Design review of the part built by this model. Coordinates are the model's own, in mm. Face numbers are marked on the shaded views. A direction names the side the tool comes from. Give positions to 0.01 mm unless a question says otherwise; leave off trailing zeros. One line per item, written item: value.
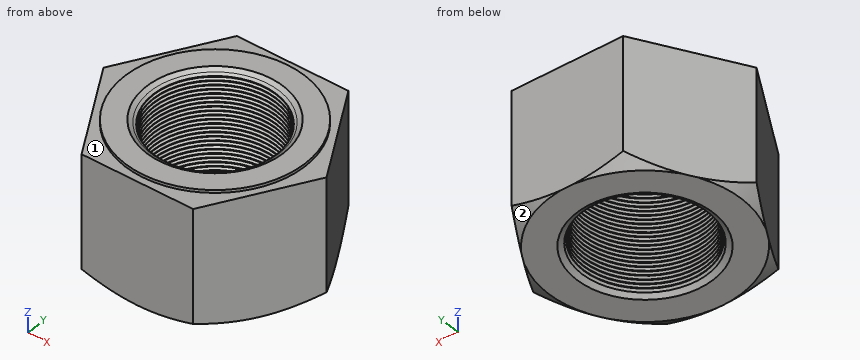
from build123d import *

# Parameters (mm, degrees)
SKETCH1_R         = 17.5
BASENUT_DEPTH     = 34.7
EXTRUDE1_START    = 0.8
SKETCH3_R         = 25.55
SKETCH3_R_2       = 17.5
EXTRUDE1_DEPTH    = 0.8
ENDCHAMFER3_SIZE  = 1.95
ENDCHAMFER3_SIZE2 = 1.125833025
LPATTERN10_COUNT  = 29
LPATTERN10_PITCH  = 1.2


with BuildPart() as part:
    # Sketch1 → BaseNut (new body)
    with BuildSketch(Plane.XY):
        Polygon((15.877132403, -27.5), (31.754264805, 0), (15.877132403, 27.5), (-15.877132403, 27.5), (-31.754264805, 0), (-15.877132403, -27.5), align=None)
        Circle(SKETCH1_R, mode=Mode.SUBTRACT)
    extrude(amount=-BASENUT_DEPTH)

    # Sketch2 → Chamfer1 (revolve, cut)
    with BuildSketch(Plane(origin=(-16.706149795, 0, -15.04811501), x_dir=(0, 0, 1), z_dir=(0, 1, 0))):
        Polygon((-19.65188499, 44.206149795), (-19.65188499, 48.460414601), (-17.195684059, 48.460414601), align=None)
    revolve(axis=Axis((0, 0, -38.770766557), (0, 0, 1)), mode=Mode.SUBTRACT)

    # Sketch6 → EndChamfer1 (revolve, cut)
    with BuildSketch(Plane(origin=(-9.197458863, 0, -10.252541137), x_dir=(0, 0, 1), z_dir=(0, 1, 0))):
        Polygon((-24.447458863, 26.697458863), (-24.447458863, 28.647458863), (-23.321625838, 26.697458863), align=None)
    revolve(axis=Axis((0, 0, 13.104863586), (0, 0, -1)), mode=Mode.SUBTRACT)

    # Sketch3 → Extrude1 (add)
    with BuildSketch(Plane(origin=(-18.48918612, 11.17895969, 0), x_dir=(1, 0, 0), z_dir=(0, 0, 1)).offset(EXTRUDE1_START)):
        with Locations((18.48918612, -11.17895969)):
            Circle(SKETCH3_R)
        with Locations((18.48918612, -11.17895969)):
            Circle(SKETCH3_R_2, mode=Mode.SUBTRACT)
    extrude(amount=-EXTRUDE1_DEPTH)

    # EndChamfer3
    endchamfer3_edges = [part.edges().sort_by_distance(p)[0] for p in [
        (-17.5, 0, 0.8),
    ]]
    endchamfer3_side = [part.faces().sort_by_distance(p)[0] for p in [
        (-24.82733687, 0, 0.8),
    ]]
    chamfer(endchamfer3_edges, length=ENDCHAMFER3_SIZE, length2=ENDCHAMFER3_SIZE2, reference=endchamfer3_side[0])

    # Sketch7 → Cut-Revolve10 (revolve, cut)
    with BuildSketch(Plane(origin=(0, 0, 0), x_dir=(1, 0, 0), z_dir=(0, 1, 0))):
        Polygon((16.5, 34.074166975), (17.5, 34.074166975), (18.366025404, 33.574166975), (17.5, 33.074166975), (16.5, 33.074166975), align=None)
    cut_revolve10 = revolve(axis=Axis((0, 0, -61.609777784), (0, 0, 1)), mode=Mode.SUBTRACT)

    # LPattern10: Cut-Revolve10 ×29
    with Locations(*[(0, 0, i * LPATTERN10_PITCH) for i in range(1, LPATTERN10_COUNT)]):
        add(cut_revolve10, mode=Mode.SUBTRACT)


solid = part.part
Item 1: Clearance check with flat-ended pins moving along their axes: P1, Ø2, axis at y = -17, z = -10.5, coming from the -X side; P2, Ø2, axis at y = -20.5, z = -17.5, coming from the -X side; P3, Ø4, axis at x = 20.5, y = 16.5, coming from the +Z side; P4, Ø6, axis at x = 25, z = -15.5, coming from the -Y side. State where each tip first meets the part, or that it passes through.
Returned:
P1: x = -22.52
P2: x = -20.5
P3: z = 0.8
P4: y = -16.89
Item 2: To check wall thickness, follow line 1 along Y through (x, z) = (0, -1.8); line 2 along X through (y, z) = (-6, -22); line 3 along X through (y, z) = (-12.5, -27.5). State the ranges of each line that lie inside material, in increasing order. Write a range as from..to.
Returned:
line 1: -27.5..-17.5, 17.5..27.5
line 2: -28.29..-16.58, 16.58..28.29
line 3: -24.54..-13.28, 13.28..24.54
Item 3: Machinability: for the marked faces 1 and 2, which of the approach directions +Z, -Z, +X, -X, +Y, -Y give a long, thin tool a straight path to every point of the face, cutting with its end or side? Answer none if there is none.
Returned:
face 1: +Z
face 2: -Z, +X, +Y
